Autodesk Inventor part; units mm, degrees
ref_plane "YZ Plane" through (0, 0, 0) normal (1, 0, 0) x (0, 1, 0)
ref_plane "XZ Plane" through (0, 0, 0) normal (0, 1, 0) x (-1, 0, 0)
ref_plane "XY Plane" through (0, 0, 0) normal (0, 0, 1) x (1, 0, 0)
sketch "Sketch1" plane through (0, 0, 0) normal (0, 0, 1) x (1, 0, 0)
  circle A0 centre (-2, 0) radius 4
  arc A1 (-2, 6) -> (-2, -6) centre (-2, 0) ccw
  circle A2 centre (-2, 0) radius 6
  line L0 (-2, -6) -> (-9, -6)
  line L1 (-9, -6) -> (-9, 6)
  line L2 (-9, 6) -> (-2, 6)
  line L3 (-2, 6) -> (-2, -6)
  point P0 (0, 0)
  point P1 (-2, -6)
  dimension "d0" = 7
extrude "Extrusion1" add sketch "Sketch1" along normal blind 5
sketch "Sketch2" plane through (0, 0, 0) normal (0, 0, -1) x (-1, 0, 0)
  circle A0 centre (2, 0) radius 4
  circle A1 centre (2, 0) radius 3.5
  point P0 (0, 0)
  dimension "d3" = 7
extrude "Extrusion2" add sketch "Sketch2" along normal blind 6 contours A1
sketch "Sketch4" plane through (-2, 0, -6) normal (0, 0, -1) x (-1, 0, 0)
  circle A0 centre (0, 0) radius 3.5
  point P0 (-2, 0)
hole "Hole1" at (-2, 0, -6) direction (0, 0, 1) diameter 3 end through all
sketch "Sketch5" plane through (-9, -6, 0) normal (0, -1, 0) x (1, 0, 0)
  circle A0 centre (-6, -1) radius 4
  circle A1 centre (-6, -1) radius 6
  line L0 (0, 0) -> (0, 5)
  line L1 (0, 5) -> (-6, 5)
  line L2 (0, 5) -> (7, 5)
  line L3 (0, 0) -> (7, 0)
  line L4 (0, 0) -> (-0.0839, 0)
  point P0 (9, 0)
  dimension "d15" = 8
  dimension "d16" = 12
  dimension "d20" = 6
extrude "Extrusion4" add sketch "Sketch5" against normal blind 5
fillet "Fillet1" radius 2 1 edges at (-9.0839, -3.5, 0)
fillet "Fillet2" radius 2 1 edges at (-9, 6, 2.5)
equation "\"d17\" = d1"
properties part number "center_holder_top_center"
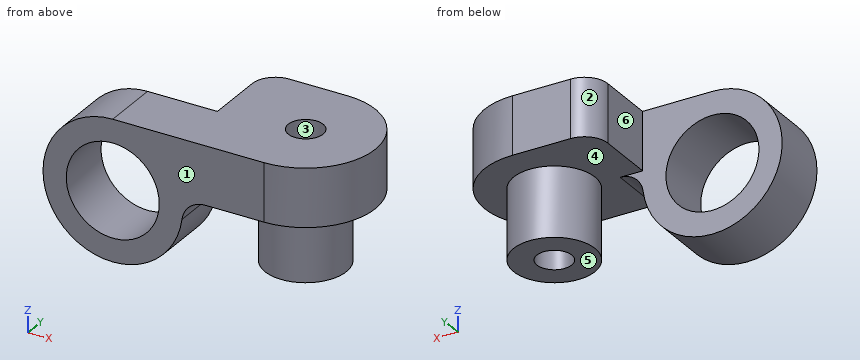
Design review of the part built by this model. Coordinates are the model's own, in mm. Face numbers are marked on the shaded views. A direction names the side the tool comes from. Round coordinates to 2 decimals unless told otherwise and drop trailing zeros. Write each loop counter-clockwise with the first axis right and the second up, starting at its lowest first coordinate (ties: lowest second). Pieces come first, ordered by that corner, then holes.
Item 1: We need section D-D on x = -13.75. Write out the cut boundary in (y, z), and give its area (3 significant figures).
Item 2: We need section C-C on z = 1. Write out the cut boundary in (x, y), and give its area (3 significant figures).
Item 3: Clearance check with flat-ended pins moving along their axes: pin 1 Ø4 at (y, z) = (0, -4.5) entering from +X; pin 2 Ø4 at (y, z) = (2.5, -0.5) entering from -X; pin 3 Ø1 at (y, z) = (1.5, 0.5) entering from +X; pin 4 Ø2 at (x, z) = (-15, 1.5) entering from -Y. State where each tip first meets the part, or that it passes through.
Item 4: For probe 1 along X at (y, z) = (0, 1.75); probe 2 along Y at (x, z) = (-2, 2.25); probe 3 along Y at (x, z) = (-15, 3.5), list the stretches that pass through material, from the lowest coordinate up.
Item 5: The part is to be moulded in two halves that separate along X. For the marked faces 1, 2 and 3, say which applies: +X half, -X half, draft (parallel to the pull), parting line (faces both ways), or undercut.
Item 6: We need section B-B on y = 0. Write out the cut boundary in (x, z), and give its area (3 significant figures).
Item 7: We need section A-A on z = -1. Write out the cut boundary in (x, y), and give its area (3 significant figures).
Item 8: For the marked faces 4, 5 and 6, list the 3-axis set-ups (+Z, -Z, +X, -X, +Y, -Y) from which the entire face can be reached by the end or side of a thin tool; tool diameter is ignored.
Returned:
1. outline: (-6, -6.87) - (-1, -6.87) - (-1, -4.8) - (-6, -4.8) - close; (-6, 2.8) - (-1, 2.8) - (-1, 5) - (-6, 5) - close
1. area: 21.3 mm2
2. outline: (-20.66, -6) - (-18.46, -6) - (-18.46, -1) - (-20.66, -1) - close; (-11.54, -6) - (-2, -6) arc R6 ccw to (-2, 6) - (-7, 6) arc R2 ccw to (-9, 4) - (-9, -1) - (-11.54, -1) - close; hole circle Ø3 at (-2, 0)
2. area: 156 mm2
3. pin 1: stops at x = 1.5
3. pin 2: stops at x = -9
3. pin 3: stops at x = 3.92
3. pin 4: passes through
4. probe 1: x = -9 to -3.5, -0.5 to 4
4. probe 2: y = -6 to -1.5, 1.5 to 6
4. probe 3: y = -6 to -1
5. face 1: draft
5. face 2: -X half
5. face 3: undercut
6. outline: (-9, 0) - (-5.5, 0) - (-5.5, -6) - (-3.5, -6) - (-3.5, 5) - (-9, 5) - close; (-0.5, -6) - (1.5, -6) - (1.5, 0) - (4, 0) - (4, 5) - (-0.5, 5) - close
6. area: 74.0 mm2
7. outline: (-21, -6) - (-19, -6) - (-19, -1) - (-21, -1) - close; (-11, -6) - (-8.79, -6) - (-8.79, -1) - (-11, -1) - close; circle Ø7 at (-2, 0); hole circle Ø3 at (-2, 0)
7. area: 52.4 mm2
8. face 4: -Z
8. face 5: -Z, +X, +Y, -Y
8. face 6: +Z, -Z, -X, +Y
